For this review, take the finished solid that the model builds, in its own axes (mm). Face numbers are marked on the shaded views. Give positions to 0.01 mm unless a question says otherwise; leave off trailing zeros. Write each loop counter-clockwise with the first axis right and the second up, starting at its lowest first coordinate (ties: lowest second). Pieces come first, ordered by that corner, then holes.
from build123d import *

# Parameters (mm, degrees)
CYLINDER_R          = 10
CYLINDER_DEPTH      = 129
CONE001_PITCH_ANGLE = 45
BOX002_W            = 5.2
BOX002_H            = 50
BOX002_DEPTH        = 126
BOX001_W            = 60
BOX001_H            = 50
BOX001_DEPTH        = 138
BOX005_W            = 4
BOX005_H            = 50
BOX005_DEPTH        = 12
BOX004_W            = 66
BOX004_H            = 50
BOX004_DEPTH        = 2
BOX006_W            = 41
BOX006_H            = 5
BOX006_DEPTH        = 12
BOX007_W            = 41
BOX007_H            = 5
BOX007_DEPTH        = 12


with BuildPart() as cylinder:
    # Cylinder → Cylinder (new body)
    with BuildSketch(Plane(origin=(-16, 59, 11), x_dir=(1, 0, 0), z_dir=(0, 0, 1))):
        Circle(CYLINDER_R)
    extrude(amount=CYLINDER_DEPTH)


with BuildPart() as cone001:
    # Cone001 → Cone001 (revolve)
    with BuildSketch(Plane.XZ):
        Polygon((0, 0), (5, 0), (12, 28), (0, 28), align=None)
    revolve(axis=Axis((0, 0, 0), (0, 0, 1)))


with BuildPart() as cone001_1:
    # Cone001 pitch: moved
    add(cone001.part.rotate(Axis((0, 0, 0), (0, 1, 0)), CONE001_PITCH_ANGLE))


with BuildPart() as cone001_2:
    # Cone001 placement: moved
    add(cone001_1.part.moved(Location((-32, 59, -2.5))))


with BuildPart() as cube002:
    # Box002 → Box002 (new body)
    with BuildSketch(Plane(origin=(-5.2, 32, -10), x_dir=(1, 0, 0), z_dir=(0, 0, 1))):
        with Locations((2.6, 25)):
            Rectangle(BOX002_W, BOX002_H)
    extrude(amount=BOX002_DEPTH)


with BuildPart() as cut002:
    # Box001 → Box001 (new body)
    with BuildSketch(Plane(origin=(-30, 32, -10), x_dir=(1, 0, 0), z_dir=(0, 0, 1))):
        with Locations((30, 25)):
            Rectangle(BOX001_W, BOX001_H)
    extrude(amount=BOX001_DEPTH)

    # Cut: cut Cube002
    add(cube002.part, mode=Mode.SUBTRACT)

    # Cut001: cut Cone001
    add(cone001_2.part, mode=Mode.SUBTRACT)

    # Cut002: cut Cylinder
    add(cylinder.part, mode=Mode.SUBTRACT)


with BuildPart() as cube005:
    # Box005 → Box005 (new body)
    with BuildSketch(Plane(origin=(-215, 176, -4), x_dir=(1, 0, 0), z_dir=(0, 0, 1))):
        with Locations((2, 25)):
            Rectangle(BOX005_W, BOX005_H)
    extrude(amount=BOX005_DEPTH)


with BuildPart() as fusion001:
    # Box004 → Box004 (new body)
    with BuildSketch(Plane(origin=(-215, 176, -4), x_dir=(1, 0, 0), z_dir=(0, 0, 1))):
        with Locations((33, 25)):
            Rectangle(BOX004_W, BOX004_H)
    extrude(amount=BOX004_DEPTH)

    # Fusion001: union Cube005
    add(cube005.part)


with BuildPart() as cube006:
    # Box006 → Box006 (new body)
    with BuildSketch(Plane(origin=(-215, 176, -4), x_dir=(1, 0, 0), z_dir=(0, 0, 1))):
        with Locations((20.5, 2.5)):
            Rectangle(BOX006_W, BOX006_H)
    extrude(amount=BOX006_DEPTH)


with BuildPart() as fusion003:
    # Box007 → Box007 (new body)
    with BuildSketch(Plane(origin=(-215, 221, -4), x_dir=(1, 0, 0), z_dir=(0, 0, 1))):
        with Locations((20.5, 2.5)):
            Rectangle(BOX007_W, BOX007_H)
    extrude(amount=BOX007_DEPTH)

    # Fusion: union Cube006
    add(cube006.part)

    # Fusion002: union Fusion001
    add(fusion001.part)


with BuildPart() as fusion003_1:
    # Fusion002 placement: moved
    add(fusion003.part.moved(Location((143.75, -144, -6))))

    # Fusion003: union Cut002
    add(cut002.part)


solid = fusion003_1.part
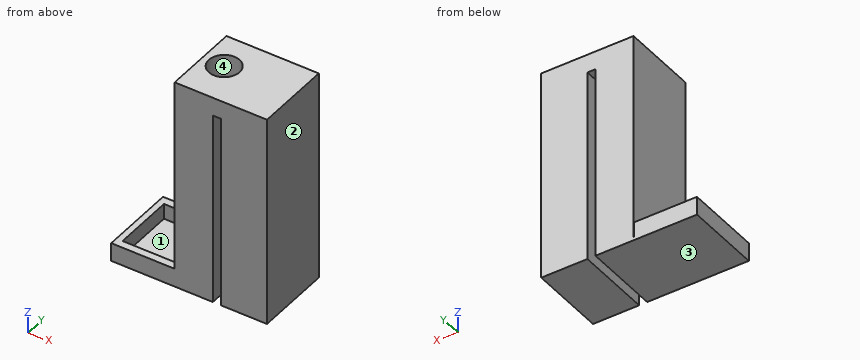
(1) We need section D-D (y = 59). Write out the cut boundary in (x, z).
(2) Clearance check with flat-ended pins moving along their axes: pin 1 Ø12 at (x, y) = (-40.5, 56.5) entering from +Z; pin 2 Ø15 at (y, z) = (45, 91) entering from -X; pin 3 Ø2.5 at (x, y) = (-3.5, 58) entering from -Z. State where each tip first meets the part, or that it passes through.
(3) The part is to be moulded in two halves that separate along X. For the marked faces 1, 2, 3 and 4, say which applies: +X half, -X half, draft (parallel to the pull), parting line (faces both ways), or undercut.
(4) We need section A-A (z = 90). Write out the cut boundary in (x, y).
(5) We need section B-B (y = 45.5). Write out the cut boundary in (x, z), and give its area (3 significant figures).
(6) We need section C-C (z = 118). Write out the cut boundary in (x, y).
(7) For L1, parallel to X at y = 59, z = 51.5; L2, parallel to X at y = 43, z = 107.5; L3, parallel to Y at x = -16, z = 89.5, list the stretches that pass through material, from the lowest coordinate up.
The answers:
1. outline: (-71.25, -10) - (-5.2, -10) - (-5.2, 7.92) - (-28.46, -6.04) - (-30, -4.5) - (-30, -8) - (-67.25, -8) - (-67.25, 2) - (-71.25, 2) - close; (-30, 10.26) - (-26, 16.93) - (-26, 128) - (-30, 128) - close; (-6, 11.1) - (-5.2, 10.3) - (-5.2, 116) - (0, 116) - (0, -10) - (30, -10) - (30, 128) - (-6, 128) - close
2. pin 1: stops at z = -8
2. pin 2: stops at x = -30
2. pin 3: stops at z = 116
3. face 1: undercut
3. face 2: +X half
3. face 3: draft
3. face 4: undercut
4. outline: (-30, 32) - (-5.2, 32) - (-5.2, 82) - (-30, 82) - close; (0, 32) - (30, 32) - (30, 82) - (0, 82) - close; hole circle Ø20 at (-16, 59)
5. outline: (-71.25, -10) - (-5.2, -10) - (-5.2, 116) - (0, 116) - (0, -10) - (30, -10) - (30, 128) - (-30, 128) - (-30, -8) - (-67.25, -8) - (-67.25, 2) - (-71.25, 2) - close
5. area: 7,750 mm2
6. outline: (-30, 32) - (30, 32) - (30, 82) - (-30, 82) - close; hole circle Ø20 at (-16, 59)
7. L1: x = -30 to -26, -6 to -5.2, 0 to 30
7. L2: x = -30 to -5.2, 0 to 30
7. L3: y = 32 to 49, 69 to 82
